Geometry: final body of the model. Coordinates: model frame, mm. A direction names the side the tool comes from. Give positions to 0.01 mm unless a question says otherwise; leave off trailing zeros. Loops run counter-clockwise (first coordinate to the right, second up) from the corner with the lowest first, then second, coordinate; pieces in that order, holes last. Notation, with made-up numbers: (19.5, 21) - (75.5, 21) arc R25 ccw to (75.5, 56) - close; hole circle Ø11 at (8, 76). An arc over 180 degrees is marked (long way). Answer in a Markdown table with one row per item.
from build123d import *

# Parameters (mm, degrees)
SKETCH1_W           = 80
SKETCH1_H           = 30
BOSS_EXTRUDE1_DEPTH = 3
SKETCH2_R           = 1.75
CUT_EXTRUDE1_DEPTH  = 3
LPATTERN1_COUNT     = 3
LPATTERN1_PITCH     = 5.5
SKETCH3_R           = 1.75
CUT_EXTRUDE2_DEPTH  = 3
SKETCH4_W           = 12
SKETCH4_H           = 31.783850417
SKETCH4_R           = 3.75
BOSS_EXTRUDE2_DEPTH = 3


with BuildPart() as part:
    # Sketch1 → Boss-Extrude1 (new body)
    with BuildSketch(Plane(origin=(0, 0, 0), x_dir=(1, 0, 0), z_dir=(0, 1, 0))):
        Rectangle(SKETCH1_W, SKETCH1_H)
    extrude(amount=BOSS_EXTRUDE1_DEPTH)

    # Sketch2 → Cut-Extrude1 (cut)
    with BuildSketch(Plane(origin=(0, 3, 0), x_dir=(1, 0, 0), z_dir=(0, 1, 0))):
        with Locations((-25, 0)):
            Circle(SKETCH2_R)
    cut_extrude1 = extrude(amount=-CUT_EXTRUDE1_DEPTH, mode=Mode.SUBTRACT)

    # LPattern1: Cut-Extrude1 ×3
    with Locations(*[(i * LPATTERN1_PITCH, 0, 0) for i in range(1, LPATTERN1_COUNT)]):
        add(cut_extrude1, mode=Mode.SUBTRACT)

    # Sketch3 → Cut-Extrude2 (cut)
    with BuildSketch(Plane(origin=(0, 3, 0), x_dir=(1, 0, 0), z_dir=(0, 1, 0))):
        with Locations((-25, -10)):
            Circle(SKETCH3_R)
        with Locations((-19.5, -10)):
            Circle(SKETCH3_R)
    cut_extrude2 = extrude(amount=-CUT_EXTRUDE2_DEPTH, mode=Mode.SUBTRACT)

    # Mirror1: Cut-Extrude2 across plane
    add(cut_extrude2.mirror(Plane.XY), mode=Mode.SUBTRACT)

    # Sketch4 → Boss-Extrude2 (add)
    with BuildSketch(Plane(origin=(0, 0, 0), x_dir=(1, 0, 0), z_dir=(0, 1, 0))):
        with Locations((-25.982178222, -30.891925209)):
            Rectangle(SKETCH4_W, SKETCH4_H)
        with Locations((-25.982178222, -40.783850417)):
            Circle(SKETCH4_R, mode=Mode.SUBTRACT)
    extrude(amount=BOSS_EXTRUDE2_DEPTH)


solid = part.part
Q1. Reachability of faces 5 (the flat face through (-1, 0, 2)), 6 (the flat face through (-36, 1, 15)), 7 (the flat face through (-19.982, 1, 31)) from +Z, -Z, +X, -X, +Y, -Y: full face, straight path, thin tool, end or side. Return the list, or none.
Check values:
| item | result |
|---|---|
| face 5 | +Z, -Z, +X, -X, -Y |
| face 6 | +Z, -X, +Y, -Y |
| face 7 | +Z, +X, +Y, -Y |
Q2. First-contact query: pin 1 (1.5 mm diameter, centred on x = -34.5, y = 2, fed in from +Z). Flat tip, straight axial feed; report the tip coordinate or a pass-through.
Check values:
| item | result |
|---|---|
| pin 1 | z = 15 |
Q3. Cut plane A-A (z = 10). Output: boundary loops of the cut face in (x, y), and give its area (3 significant figures).
Check values:
| item | result |
|---|---|
| outline | (-40, 0) - (-26.75, 0) - (-26.75, 3) - (-40, 3) - close; (-23.25, 0) - (-21.25, 0) - (-21.25, 3) - (-23.25, 3) - close; (-17.75, 0) - (40, 0) - (40, 3) - (-17.75, 3) - close |
| area | 219 mm² |
Q4. Cut plane C-C (x = -25). Output: boundary loops of the cut face in (y, z).
Check values:
| item | result |
|---|---|
| outline | (0, -15) - (3, -15) - (3, -11.75) - (0, -11.75) - close; (0, -8.25) - (3, -8.25) - (3, -1.75) - (0, -1.75) - close; (0, 1.75) - (3, 1.75) - (3, 8.25) - (0, 8.25) - close; (0, 11.75) - (3, 11.75) - (3, 37.16) - (0, 37.16) - close; (0, 44.4) - (3, 44.4) - (3, 46.78) - (0, 46.78) - close |
Q5. Cut plane D-D (y = 1.35). Give the number of separate pieces and of enclosed holes in the cut face, and give its area (3 significant figures).
Check values:
| item | result |
|---|---|
| separate pieces | 1 |
| enclosed holes | 8 |
| area | 2,670 mm² |
Q6. Draft query along X for faces 1 (the flat face through (-31.982, 1, 31)), 2 (the cylindrical face through (-20.79, 1.52, -8.82)), 3 (the flat face through (40, 1, 0)), 4 (the flat face through (10, 1, 15)). Return one class per face: pulls with the +X half, pulls with the -X half, needs draft (parallel to the pull), parting line crosses it, or undercut.
Check values:
| item | result |
|---|---|
| face 1 | pulls with the -X half |
| face 2 | undercut |
| face 3 | pulls with the +X half |
| face 4 | needs draft |
Q7. Cut plane B-B (x = -14). Output: boundary loops of the cut face in (y, z).
Check values:
| item | result |
|---|---|
| outline | (0, -15) - (3, -15) - (3, -1.75) - (0, -1.75) - close; (0, 1.75) - (3, 1.75) - (3, 15) - (0, 15) - close |
Q8. Material intervals for line 1 along X through (y, z) = (1.05, 10); line 2 along Z through (x, y) = (-14, 1.2); line 3 along X through (y, z) = (0.8, 0), sorted ascending.
Check values:
| item | result |
|---|---|
| line 1 | -40 to -26.75, -23.25 to -21.25, -17.75 to 40 |
| line 2 | -15 to -1.75, 1.75 to 15 |
| line 3 | -40 to -26.75, -23.25 to -21.25, -17.75 to -15.75, -12.25 to 40 |
